Input: part model. Units: mm. Frame: model coordinates. A direction names the side the tool comes from. Coordinates: 2 decimals unless noted, no trailing zeros. Use one line per item in the form item = value. Start each with the question number.
(1) Cut plane A-A on x = 0. State how many separate pieces and enclosed holes the cut face has, plus the area to 3 significant figures.
(2) First-contact query: pin 1 (14.5 mm diameter, centred on x = -19.02, y = 6.18, fed in from -Z); pin 2 (5 mm diameter, centred on x = 15.5, y = -3, fed in from -Z); pin 3 (18.5 mm diameter, centred on x = 12.5, y = -1, fed in from +Z); pin 4 (1 mm diameter, centred on y = 6.5, z = 1, fed in from -X). Flat tips, straight axial feed; report the tip coordinate or a pass-through.
(3) Ray query, line 1 along Y through (x, z) = (0, 1); line 2 along X through (y, z) = (-20, 1.4); line 3 along Y through (x, z) = (19, 0.2). Return the intervals inside material, ascending.
(4) Pull-direction query (X, two-part tool) for faces 3 (the face through (7, 0, 0)), 4 (the face through (6, 0, 2)); classes: released by +X, released by -X, zero draft, split by the parting line, or undercut.
(5) Set-up query: faces 1 (the face through (27.6, 8.9, 1)), 2 (the face through (18.559, -24.204, 2.986)). Return all of +Z, -Z, +X, -X, +Y, -Y with unobstructed straight access to the full face (end or side cutting, diameter ignored); none if empty.
```python
from build123d import *

# Parameters (mm, degrees)
F0_R     = 9
F0_R_2   = 1.5
F3_DEPTH = 25
F4_SIZE  = 0.99999


# Not quite as in the source:
# - a fillet or chamfer is up to 0.001 mm smaller than in the source, because OpenCascade refuses the exact size


with BuildPart() as f2:
    # F1 (on Right) → F2 (revolve)
    with BuildSketch(Plane.YZ):
        Polygon((0, 2), (0, 0), (35.5, 0), (35.5, 1), (34.9226497308, 2), (35.5, 3), (35.5, 4), (30.5, 4), (30.5, 2), align=None)
    revolve(axis=Axis((0, 0, 11.7082232609), (0, 0, 1)))

    # F0 (on Top) → F3 (cut)
    with BuildSketch(Plane.XY):
        with Locations((11.7557050458, -16.1803398875)):
            Circle(F0_R)
        with Locations((-11.7557050458, -16.1803398875)):
            Circle(F0_R)
        with Locations((-19.0211303259, 6.1803398875)):
            Circle(F0_R)
        with Locations((0, 20)):
            Circle(F0_R)
        with Locations((19.0211303259, 6.1803398875)):
            Circle(F0_R)
        Circle(F0_R_2)
    extrude(amount=F3_DEPTH, mode=Mode.SUBTRACT)

    # F4 (size 1 in the source; OpenCascade refuses exactly that, so slightly less here)
    f4_edges = [f2.edges().sort_by_distance(p)[0] for p in [
        (0, -35.5, 4),
        (0, -35.5, 0),
    ]]
    chamfer(f4_edges, length=F4_SIZE)


solid = f2.part
```
Values:
q1.separate_pieces = 3
q1.enclosed_holes = 0
q1.area = 117 mm2
q2.pin_1 = through
q2.pin_2 = 0
q2.pin_3 = 2
q2.pin_4 = -34.99
q3.line_1 = -35.5 to -1.5, 1.5 to 11, 29 to 35.5
q3.line_2 = -29.05 to -19.9, -3.61 to 3.61, 19.9 to 29.05
q3.line_3 = -29.04 to -21.52, -10.84 to -2.82, 15.18 to 29.04
q4.face_3 = zero draft
q4.face_4 = undercut
q5.face_1 = +Z, -Z
q5.face_2 = +Z
